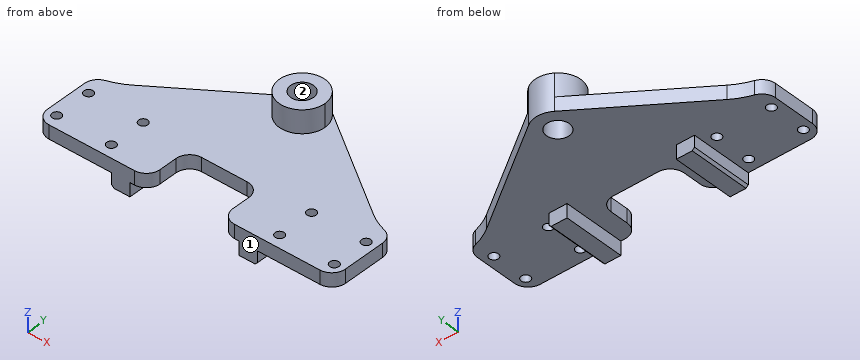
```python
from build123d import *

# Parameters (mm, degrees)
SKETCH_1_W          = 4
SKETCH_1_H          = 13.5
EXTRUDE_1_DEPTH     = 3
EXTRUDE_1_2_DEPTH   = 3
EXTRUDE_1_3_DEPTH   = 3
EXTRUDE_1_4_DEPTH   = 3
SKETCH_2_R          = 2.5
EXTRUDE_2_DEPTH     = 3
FILLET_3_R          = 3
FILLET_4_R          = 5
CHAMFER_1_SIZE      = 0.5
SKETCH_5_R          = 1
CUT_EXTRUDE_3_DEPTH = 4
CUT_EXTRUDE_START   = -14
CUT_EXTRUDE_4_DEPTH = 14
FILLET_6_R          = 3
SKETCH_10_R         = 2.5
EXTRUDE_5_DEPTH     = 5


with BuildPart() as part:
    # Sketch 1 → Extrude 1 (new body)
    with BuildSketch(Plane.XY):
        with Locations((-35, -41.75)):
            Rectangle(SKETCH_1_W, SKETCH_1_H)
    extrude(amount=EXTRUDE_1_DEPTH)



with BuildPart() as body_2:
    # Sketch 1 → Extrude 1 2 (new body)
    with BuildSketch(Plane.XY):
        with Locations((-14, -41.75)):
            Rectangle(SKETCH_1_W, SKETCH_1_H)
    extrude(amount=EXTRUDE_1_2_DEPTH)


with BuildPart() as body_3:
    # Sketch 1 → Extrude 1 3 (new body)
    with BuildSketch(Plane.XY):
        with Locations((14, -41.75)):
            Rectangle(SKETCH_1_W, SKETCH_1_H)
    extrude(amount=EXTRUDE_1_3_DEPTH)


with BuildPart() as body_4:
    # Sketch 1 → Extrude 1 4 (new body)
    with BuildSketch(Plane.XY):
        with Locations((35, -41.75)):
            Rectangle(SKETCH_1_W, SKETCH_1_H)
    extrude(amount=EXTRUDE_1_4_DEPTH)


with BuildPart() as part_1:
    add(part.part)

    add(body_2.part)  # Extrude 2 merges body 2

    add(body_3.part)  # Extrude 2 merges body 3

    add(body_4.part)  # Extrude 2 merges body 4
    # Sketch 2 → Extrude 2 (add)
    with BuildSketch(Plane.XY.offset(3)):
        with BuildLine():
            Line((-37, -35), (-37, -48.5))
            Line((-37, -48.5), (-12, -48.5))
            Line((-12, -48.5), (-8, -48.5))
            Line((-8, -48.5), (-8, -38.5))
            Line((-8, -38.5), (8, -38.5))
            Line((8, -38.5), (8, -48.5))
            Line((8, -48.5), (12, -48.5))
            Line((12, -48.5), (37, -48.5))
            Line((37, -48.5), (37, -35))
            Line((37, -35), (37, -34))
            Line((37, -34), (35, -34))
            ThreePointArc((35, -34), (30.508154972, -33.311650088), (26.428571429, -31.3097771))
            Line((26.428571429, -31.3097771), (2.857142857, -14.896740967))
            ThreePointArc((2.857142857, -14.896740967), (0, -14), (-2.857142857, -14.896740967))
            Line((-2.857142857, -14.896740967), (-26.428571429, -31.3097771))
            ThreePointArc((-26.428571429, -31.3097771), (-30.508154972, -33.311650088), (-35, -34))
            Line((-35, -34), (-37, -34))
            Line((-37, -34), (-37, -35))
        make_face()
        with Locations((0, -19)):
            Circle(SKETCH_2_R, mode=Mode.SUBTRACT)
    extrude(amount=EXTRUDE_2_DEPTH)

    # Fillet 3
    fillet_3_edges = [part_1.edges().sort_by_distance(p)[0] for p in [
        (-8, -48.5, 4.5),
        (-8, -38.5, 4.5),
        (8, -38.5, 4.5),
        (8, -48.5, 4.5),
        (37, -48.5, 3),
        (-37, -48.5, 3),
    ]]
    fillet(fillet_3_edges, radius=FILLET_3_R)

    # Fillet 4
    # the kernel refuses this fillet: 5 mm, written as the material it takes off along each edge
    with BuildSketch(Plane(origin=(37, -34, -8.934299833), x_dir=(0, -1, 0), z_dir=(0, 0, 1))) as fillet_4_piece_1:
        with BuildLine():
            CenterArc((4.773719933, -5), FILLET_4_R, 90, 81.373073441)
            Line((-0.16971005, -4.25), (-0.664053048, -4.175))
            ThreePointArc((-0.664053048, -4.175), (-0.5, -2), (-0.5, 0))
            Line((-0.5, 0), (0, 0.5))
            Line((0, 0.5), (4.773719933, 0.5))
            Line((4.773719933, 0.5), (4.773719933, 0))
        make_face()
    extrude(amount=26.868599666, mode=Mode.SUBTRACT)
    with BuildSketch(Plane(origin=(-37, -34, -8.934299833), x_dir=(0.9992036788156995, 0.039899977959549054, 0), z_dir=(0, 0, 1))) as fillet_4_piece_2:
        with BuildLine():
            CenterArc((4.805547074, -4.969418409), FILLET_4_R, 96.340219202, 81.373073441)
            Line((-0.19047132, -4.769918519), (-0.69007316, -4.74996853))
            Line((-0.69007316, -4.74996853), (-0.499601839, 0.019949989))
            Line((-0.499601839, 0.019949989), (0.019949989, 0.499601839))
            ThreePointArc((0.019949989, 0.499601839), (2.018357347, 0.419801883), (4.198171061, 0.496941841))
            Line((4.198171061, 0.496941841), (4.253387062, 0))
        make_face()
    extrude(amount=26.868599666, mode=Mode.SUBTRACT)

    # Chamfer 1
    chamfer_1_edges = [part_1.edges().sort_by_distance(p)[0] for p in [
        (-16, -41.75, 0),
        (-33, -41.75, 0),
        (16, -41.75, 0),
        (33, -41.75, 0),
    ]]
    chamfer(chamfer_1_edges, length=CHAMFER_1_SIZE)

    # Sketch 5 → Cut-Extrude 3 (cut)
    with BuildSketch(Plane.XY.offset(6)):
        with Locations((-18.5, -45.75)):
            Circle(SKETCH_5_R)
        with Locations((-18.5, -37.75)):
            Circle(SKETCH_5_R)
        with Locations((-30.5, -45.75)):
            Circle(SKETCH_5_R)
        with Locations((-30.5, -37.75)):
            Circle(SKETCH_5_R)
        with Locations((18.5, -45.75)):
            Circle(SKETCH_5_R)
        with Locations((18.5, -37.75)):
            Circle(SKETCH_5_R)
        with Locations((30.5, -45.75)):
            Circle(SKETCH_5_R)
        with Locations((30.5, -37.75)):
            Circle(SKETCH_5_R)
    extrude(amount=-CUT_EXTRUDE_3_DEPTH, mode=Mode.SUBTRACT)

    # Sketch 9 → Cut-Extrude 4 (cut)
    with BuildSketch(Plane.XY.offset(6).offset(CUT_EXTRUDE_START)):
        with BuildLine():
            Line((37, -45.5), (37, -38.773719933))
            ThreePointArc((37, -38.773719933), (35.791437722, -35.514118731), (32.75, -33.83028995))
            Line((32.75, -33.83028995), (32.75, -48.5))
            Line((32.75, -48.5), (34, -48.5))
            ThreePointArc((34, -48.5), (36.121320344, -47.621320344), (37, -45.5))
        make_face()
        with BuildLine():
            Line((-32.75, -33.83028995), (-32.75, -48.5))
            Line((-32.75, -48.5), (-34, -48.5))
            ThreePointArc((-34, -48.5), (-36.121320344, -47.621320344), (-37, -45.5))
            Line((-37, -45.5), (-37, -38.773719933))
            ThreePointArc((-37, -38.773719933), (-35.791437722, -35.514118731), (-32.75, -33.83028995))
        make_face()
    extrude(amount=CUT_EXTRUDE_4_DEPTH, mode=Mode.SUBTRACT)

    # Fillet 6
    fillet_6_edges = [part_1.edges().sort_by_distance(p)[0] for p in [
        (32.75, -33.83028995, 4.5),
        (-32.75, -33.83028995, 4.5),
        (32.75, -48.5, 4.5),
        (-32.75, -48.5, 4.5),
    ]]
    fillet(fillet_6_edges, radius=FILLET_6_R)

    # Sketch 10 → Extrude 5 (add)
    with BuildSketch(Plane.XY.offset(6)):
        with BuildLine():
            ThreePointArc((5, -19), (4.432026302, -16.685449751), (2.857142857, -14.896740967))
            ThreePointArc((2.857142857, -14.896740967), (0, -14), (-2.857142857, -14.896740967))
            ThreePointArc((-2.857142857, -14.896740967), (-2.314550249, -23.432026302), (5, -19))
        make_face()
        with Locations((0, -19)):
            Circle(SKETCH_10_R, mode=Mode.SUBTRACT)
    extrude(amount=EXTRUDE_5_DEPTH)


solid = part_1.part
```
The listing builds one solid part. Answer for the finished solid, in the listing's coordinates (mm). Face numbers are marked on the shaded views. Coordinates: 2 decimals unless noted, no trailing zeros. Loops run counter-clockwise (first coordinate to the right, second up) from the corner with the lowest first, then second, coordinate; pieces in that order, holes last. Notation, with made-up numbers: M -22,59 L 16,59 A6 ccw 16,63 Z; hole C -35.75,-22.5 d1. An arc over 180 degrees is marked long. Answer as CSV lines item,"result". Start each with the question number.
(1) The part is cut by section D-D (x = -18.5). Give the vertices of the cut face in (y, z).
(2) The part is cut by section A-A (y = -37.75). State how many separate pieces and enclosed holes the cut face has, and give its area (3 significant figures).
(3) The part is cut by section C-C (x = 0). Give the vertices of the cut face in (y, z), and give its area (3 significant figures).
(4) The mould has two halves that part along X. Classify the marked faces 1 and 2: pulls with the +X half, pulls with the -X half, needs draft (parallel to the pull), parting line crosses it, or undercut.
(5) Find the intervals of material crossed by L1, parallel to X at y = -46, z = 2; L2, parallel to Y at x = 18.5, z = 4.45; L3, parallel to Y at x = -30.5, z = 4, in increasing order. Write a range as [from, to].
(6) Given pin 1 (2.5 mm diameter, centred on x = 18.5, y = -37.75, fed in from +Z); pin 2 (1.3 mm diameter, centred on y = -45, z = 1.5, fed in from -X); pin 3 (2.5 mm diameter, centred on x = 30.5, y = -37.75, fed in from -Z); pin 4 (1.2 mm diameter, centred on x = 18.5, y = -45.75, fed in from -Z), each flat-ended and moving along its own axis, determine where each tip first touches the part or whether it passes through.
Determined:
1,outline,"M -48.5,3 L -46.75,3 L -46.75,6 L -48.5,6 Z; M -44.75,3 L -38.75,3 L -38.75,6 L -44.75,6 Z; M -36.75,3 L -25.79,3 L -25.79,6 L -36.75,6 Z"
2,separate pieces,"5"
2,enclosed holes,"0"
2,area,"196 mm2"
3,outline,"M -38.5,3 L -21.5,3 L -21.5,11 L -24,11 L -24,6 L -38.5,6 Z; M -16.5,3 L -14,3 L -14,11 L -16.5,11 Z"
3,area,"83.5 mm2"
4,face 1,"needs draft"
4,face 2,"undercut"
5,L1,"[-16, -12], [12, 16]"
5,L2,"[-48.5, -46.75], [-44.75, -38.75], [-36.75, -25.79]"
5,L3,"[-48.4, -46.75], [-44.75, -38.75], [-36.75, -33.31]"
6,pin 1,"z = 6"
6,pin 2,"x = -16"
6,pin 3,"z = 3"
6,pin 4,"through"
